The listing builds one solid part. Answer for the finished solid, in the listing's coordinates (mm). Face numbers are marked on the shaded views. A direction names the side the tool comes from. Round coordinates to 2 decimals unless told otherwise and drop trailing zeros. Loops run counter-clockwise (first coordinate to the right, second up) from the corner with the lowest first, then second, coordinate; pieces in that order, holes last. Notation, with made-up numbers: M 32.5,19.5 L 80.5,19.5 A15 cw 80.5,42.5 Z; hole C 3.5,86.5 d8. An arc over 180 degrees is marked long. Put each result on its own line as item: value. Start each with the question number.
(1) Flat-ended cylindrical pins translate along their axes: P1, Ø7.5, axis at x = -2, z = 2.5, coming from the -Y side; P2, Ø6, axis at x = -4.5, z = -4.5, coming from the -Y side; P3, Ø2, axis at x = -3, y = 20.5, coming from the -Z side; P4, Ø5, axis at y = 16.5, z = 5.5, coming from the +X side. Find the tip coordinate at first contact, or state that the pin passes through.
(2) Which of the six approach directions +Z, -Z, +X, -X, +Y, -Y give full straight-line access (tool end or side, diameter ignored) to the marked faces 4 and 5?
(3) Section A-A, the plane x = 0 is taken. Determine the outline of the cut face in (y, z), then the cut area to 3 significant figures.
(4) Straight lines are drawn through the part: line 1 (X direction, y = 26, z = 0); line 2 (Y direction, x = 4.75, z = 2); line 3 (Y direction, x = 1.75, z = 2.75). For each, find the intervals that lie inside material, in ascending order.
(5) Determine the mould class of the marked faces 1, 2 and 3 for opening direction Z: released by +Z, released by -Z, zero draft, split by the parting line, or undercut.
(6) Section C-C, the plane y = 21.5 is taken. Determine the outline of the cut face in (x, z), then the cut area to 3 significant figures.
(7) Section B-B, the plane z = 0 is taken. Determine the outline of the cut face in (x, y), then the cut area to 3 significant figures.
(8) Section D-D, the plane y = 3.75 is taken. Determine the outline of the cut face in (x, z).
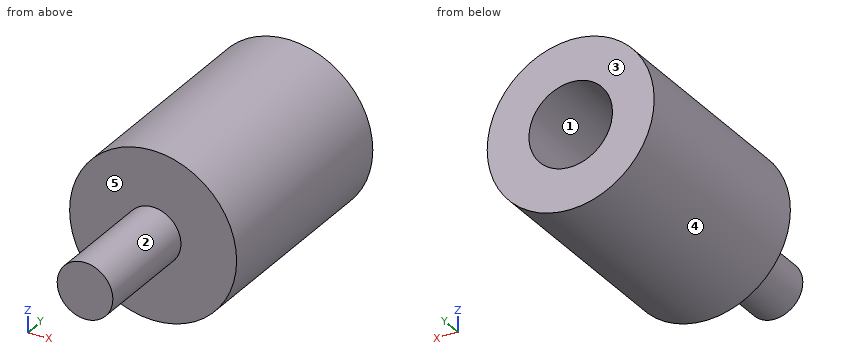
```python
from build123d import *

# Parameters (mm, degrees)
SKETCH1_R           = 2.5
BOSS_EXTRUDE2_DEPTH = 10
SKETCH2_R           = 7.5
BOSS_EXTRUDE3_DEPTH = 20
SKETCH3_R           = 3.75
CUT_EXTRUDE1_DEPTH  = 14


with BuildPart() as part:
    # Sketch1 → Boss-Extrude2 (new body)
    with BuildSketch(Plane(origin=(0, 0, 0), x_dir=(1, 0, 0), z_dir=(0, 1, 0))):
        with Locations(Location((0, 0, 0), (0, 0, 270))):  # turned: the seam where the file's is
            Circle(SKETCH1_R)
    extrude(amount=BOSS_EXTRUDE2_DEPTH)

    # Sketch2 → Boss-Extrude3 (add)
    with BuildSketch(Plane(origin=(0, 10, 0), x_dir=(1, 0, 0), z_dir=(0, 1, 0))):
        with Locations(Location((0, 0, 0), (0, 0, 270))):  # turned: the seam where the file's is
            Circle(SKETCH2_R)
    extrude(amount=BOSS_EXTRUDE3_DEPTH)

    # Sketch3 → Cut-Extrude1 (cut)
    with BuildSketch(Plane(origin=(0, 30, 0), x_dir=(1, 0, 0), z_dir=(0, 1, 0))):
        with Locations(Location((0, 0, 0), (0, 0, 270))):  # turned: the seam where the file's is
            Circle(SKETCH3_R)
    extrude(amount=-CUT_EXTRUDE1_DEPTH, mode=Mode.SUBTRACT)


solid = part.part
```
Recorded:
1. P1: stops at y = 0
1. P2: stops at y = 10
1. P3: stops at z = -7.23
1. P4: stops at x = 6.87
2. face 4: +Y, -Y
2. face 5: -Y
3. outline: M 0,-2.5 L 10,-2.5 L 10,-7.5 L 30,-7.5 L 30,-3.75 L 16,-3.75 L 16,3.75 L 30,3.75 L 30,7.5 L 10,7.5 L 10,2.5 L 0,2.5 Z
3. area: 245 mm²
4. line 1: x = -7.5 to -3.75, 3.75 to 7.5
4. line 2: y = 10 to 30
4. line 3: y = 10 to 16
5. face 1: undercut
5. face 2: split by the parting line
5. face 3: zero draft
6. outline: C 0,0 d15; hole C 0,0 d7.5
6. area: 133 mm²
7. outline: M -7.5,10 L -2.5,10 L -2.5,0 L 2.5,0 L 2.5,10 L 7.5,10 L 7.5,30 L 3.75,30 L 3.75,16 L -3.75,16 L -3.75,30 L -7.5,30 Z
7. area: 245 mm²
8. outline: C 0,0 d5
